CAD build for the part. Positions are in the model's coordinates, mm. A direction names the side the tool comes from. Coordinates: 2 decimals unless noted, no trailing zeros. Answer in a Markdown table with one row per item. Add a question column.
Q1. Drill centre lines: line 1 along Y through (x, z) = (-4.5, 24); line 2 along Y through (x, z) = (6, 70); line 3 along X through (y, z) = (-6, 15). Where is each one in solid material? Low to high. Write a range as from..to.
Q2. 3-axis set-ups, long thin cutter, end or side, ignore diameter. For faces 1 (the cylindrical face through (-20, -15, 40)), 2 (the cylindrical face through (0, 15, 30)), 3 (the cylindrical face through (0, -15, 30)), 4 (the cylindrical face through (-10, 0, 13)): which of +Z, -Z, +X, -X, +Y, -Y reach the whole face in a straight line?
Q3. Pin check, flat tips, straight feed: pin 1 (2 mm diameter, centred on y = 0, z = 53.5, fed in from -X); pin 2 (1 mm diameter, centred on y = 10, z = 56, fed in from -X); pin 3 (5 mm diameter, centred on y = -18.5, z = 54, fed in from -X). Stop position of each tip, or through.
```python
from build123d import *

# Parameters (mm, degrees)
F0_R         = 10
F1_DEPTH     = 25
F2_W         = 50
F2_H         = 50
F3_DEPTH     = 50
F4_T1_DEPTH  = 87.4998500005
F4_T3_DEPTH  = 0.0002
F4_T5_DEPTH  = 0.0002
F4_S9_W      = 25.5
F4_S9_H      = 25.5
F4_T10_DEPTH = 25.5
F4_S15_W     = 25.5
F4_S15_H     = 25.5
F4_T16_DEPTH = 25.5
F4_S21_W     = 25.5
F4_S21_H     = 25.5
F4_T22_DEPTH = 25.5
F4_S27_W     = 25.5
F4_S27_H     = 25.5
F4_T28_DEPTH = 25.5
F4_T34_DEPTH = 174.999500001
F4_S35_R     = 10
F4_T36_DEPTH = 91
F4_T40_DEPTH = 174.999500001
F4_S41_R     = 10
F4_T42_DEPTH = 91


# Not quite as in the source:
# - a fillet or chamfer that OpenCascade refuses, or shapes differently, is made with other operations: its cross-section is extruded or revolved along the edge and cut away or added


with BuildPart() as f1:
    # F0 (on Top) → F1 (new body)
    with BuildSketch(Plane.XY):
        Circle(F0_R)
    extrude(amount=F1_DEPTH)

    # F2 (on face) → F3 (join)
    with BuildSketch(Plane.XY.offset(25)):
        Rectangle(F2_W, F2_H)
    extrude(amount=F3_DEPTH)

    # F4: fillet of radius 25 on 10 edges, made by hand

    # F4_s2 → F4_t1 (cut)
    with BuildSketch(Plane.XY.offset(-37.4997500005)):
        with BuildLine():
            ThreePointArc((-0.0001, -25.0001), (-17.6777695297, -17.6777695297), (-25.0001, -0.0001))
            Line((-25.0001, -0.0001), (-25.5001, -0.0001))
            ThreePointArc((-25.5001, -0.0001), (-25.5, -12.50005), (-25.5, -25))
            Line((-25.5, -25), (-25, -25.5))
            ThreePointArc((-25, -25.5), (-12.50005, -25.5), (-0.0001, -25.5001))
            Line((-0.0001, -25.5001), (-0.0001, -25.0001))
        make_face()
        with BuildLine():
            ThreePointArc((25.0001, -0.0001), (17.6777695297, -17.6777695297), (0.0001, -25.0001))
            Line((0.0001, -25.0001), (0.0001, -25.5001))
            ThreePointArc((0.0001, -25.5001), (12.50005, -25.5), (25, -25.5))
            Line((25, -25.5), (25.5, -25))
            ThreePointArc((25.5, -25), (25.5, -12.50005), (25.5001, -0.0001))
            Line((25.5001, -0.0001), (25.0001, -0.0001))
        make_face()
        with BuildLine():
            ThreePointArc((25.0001, 0.0001), (17.6777695297, 17.6777695297), (0.0001, 25.0001))
            Line((0.0001, 25.0001), (0.0001, 25.5001))
            ThreePointArc((0.0001, 25.5001), (12.50005, 25.5), (25, 25.5))
            Line((25, 25.5), (25.5, 25))
            ThreePointArc((25.5, 25), (25.5, 12.50005), (25.5001, 0.0001))
            Line((25.5001, 0.0001), (25.0001, 0.0001))
        make_face()
        with BuildLine():
            ThreePointArc((-0.0001, 25.0001), (-17.6777695297, 17.6777695297), (-25.0001, 0.0001))
            Line((-25.0001, 0.0001), (-25.5001, 0.0001))
            ThreePointArc((-25.5001, 0.0001), (-25.5, 12.50005), (-25.5, 25))
            Line((-25.5, 25), (-25, 25.5))
            ThreePointArc((-25, 25.5), (-12.50005, 25.5), (-0.0001, 25.5001))
            Line((-0.0001, 25.5001), (-0.0001, 25.0001))
        make_face()
    extrude(amount=F4_T1_DEPTH, mode=Mode.SUBTRACT)

    # F4_s4 → F4_t3 (cut)
    with BuildSketch(Plane.YZ.offset(-0.0001)):
        with BuildLine():
            ThreePointArc((-25.0001, 50.0001), (-17.6777695297, 67.6777695297), (-0.0001, 75.0001))
            Line((-0.0001, 75.0001), (-0.0001, 75.5001))
            ThreePointArc((-0.0001, 75.5001), (-12.50005, 75.5), (-25, 75.5))
            Line((-25, 75.5), (-25.5, 75))
            ThreePointArc((-25.5, 75), (-25.5, 62.50005), (-25.5001, 50.0001))
            Line((-25.5001, 50.0001), (-25.0001, 50.0001))
        make_face()
        with BuildLine():
            ThreePointArc((25.0001, 50.0001), (17.6777695297, 67.6777695297), (0.0001, 75.0001))
            Line((0.0001, 75.0001), (0.0001, 75.5001))
            ThreePointArc((0.0001, 75.5001), (12.50005, 75.5), (25, 75.5))
            Line((25, 75.5), (25.5, 75))
            ThreePointArc((25.5, 75), (25.5, 62.50005), (25.5001, 50.0001))
            Line((25.5001, 50.0001), (25.0001, 50.0001))
        make_face()
    extrude(amount=F4_T3_DEPTH, mode=Mode.SUBTRACT)

    # F4_s6 → F4_t5 (cut)
    with BuildSketch(Plane.XZ.offset(-0.0001)):
        with BuildLine():
            ThreePointArc((25.0001, 50.0001), (17.6777695297, 67.6777695297), (0.0001, 75.0001))
            Line((0.0001, 75.0001), (0.0001, 75.5001))
            ThreePointArc((0.0001, 75.5001), (12.50005, 75.5), (25, 75.5))
            Line((25, 75.5), (25.5, 75))
            ThreePointArc((25.5, 75), (25.5, 62.50005), (25.5001, 50.0001))
            Line((25.5001, 50.0001), (25.0001, 50.0001))
        make_face()
        with BuildLine():
            ThreePointArc((-0.0001, 75.0001), (-17.6777695297, 67.6777695297), (-25.0001, 50.0001))
            Line((-25.0001, 50.0001), (-25.5001, 50.0001))
            ThreePointArc((-25.5001, 50.0001), (-25.5, 62.50005), (-25.5, 75))
            Line((-25.5, 75), (-25, 75.5))
            ThreePointArc((-25, 75.5), (-12.50005, 75.5), (-0.0001, 75.5001))
            Line((-0.0001, 75.5001), (-0.0001, 75.0001))
        make_face()
    extrude(amount=F4_T5_DEPTH, mode=Mode.SUBTRACT)


with BuildPart() as f4_tool8:
    # F4_s9 → F4_t10 (new body)
    with BuildSketch(Plane.XZ.offset(0.0001)):
        with Locations((-12.7501, 62.7501)):
            Rectangle(F4_S9_W, F4_S9_H)
    extrude(amount=F4_T10_DEPTH)

    # F4_s11 → F4_t12 (revolve, cut)
    with BuildSketch(Plane(origin=(-0.0001, -0.0001, 50.0001), x_dir=(0.7071067812, 0, -0.7071067812), z_dir=(-0.7071067812, 0, -0.7071067812))):
        with BuildLine():
            ThreePointArc((0, -25), (25, 0), (0, 25))
            Line((0, 25), (0, -25))
        make_face()
    revolve(axis=Axis((-0.0001, -0.0001, 50.0001), (0, -1, 0)), mode=Mode.SUBTRACT)


with BuildPart() as f1_1:
    add(f1.part)

    # F4_t7: cut F4_tool8
    add(f4_tool8.part, mode=Mode.SUBTRACT)


with BuildPart() as f4_tool14:
    # F4_s15 → F4_t16 (new body)
    with BuildSketch(Plane.YZ.offset(0.0001)):
        with Locations((-12.7501, 62.7501)):
            Rectangle(F4_S15_W, F4_S15_H)
    extrude(amount=F4_T16_DEPTH)

    # F4_s17 → F4_t18 (revolve, cut)
    with BuildSketch(Plane(origin=(0.0001, -0.0001, 50.0001), x_dir=(0, 0.7071067812, -0.7071067812), z_dir=(0, -0.7071067812, -0.7071067812))):
        with BuildLine():
            ThreePointArc((0, -25), (25, 0), (0, 25))
            Line((0, 25), (0, -25))
        make_face()
    revolve(axis=Axis((0.0001, -0.0001, 50.0001), (1, 0, 0)), mode=Mode.SUBTRACT)


with BuildPart() as f1_2:
    add(f1_1.part)

    # F4_t13: cut F4_tool14
    add(f4_tool14.part, mode=Mode.SUBTRACT)


with BuildPart() as f4_tool20:
    # F4_s21 → F4_t22 (new body)
    with BuildSketch(Plane.YZ.offset(0.0001)):
        with Locations((12.7501, 62.7501)):
            Rectangle(F4_S21_W, F4_S21_H)
    extrude(amount=F4_T22_DEPTH)

    # F4_s23 → F4_t24 (revolve, cut)
    with BuildSketch(Plane(origin=(0.0001, 0.0001, 50.0001), x_dir=(0, -0.7071067812, -0.7071067812), z_dir=(0, -0.7071067812, 0.7071067812))):
        with BuildLine():
            ThreePointArc((0, -25), (25, 0), (0, 25))
            Line((0, 25), (0, -25))
        make_face()
    revolve(axis=Axis((0.0001, 0.0001, 50.0001), (1, 0, 0)), mode=Mode.SUBTRACT)


with BuildPart() as f1_3:
    add(f1_2.part)

    # F4_t19: cut F4_tool20
    add(f4_tool20.part, mode=Mode.SUBTRACT)


with BuildPart() as f4_tool26:
    # F4_s27 → F4_t28 (new body)
    with BuildSketch(Plane.XZ.offset(-0.0001)):
        with Locations((-12.7501, 62.7501)):
            Rectangle(F4_S27_W, F4_S27_H)
    extrude(amount=-F4_T28_DEPTH)

    # F4_s29 → F4_t30 (revolve, cut)
    with BuildSketch(Plane(origin=(-0.0001, 0.0001, 50.0001), x_dir=(0.7071067812, 0, -0.7071067812), z_dir=(0.7071067812, 0, 0.7071067812))):
        with BuildLine():
            ThreePointArc((0, -25), (25, 0), (0, 25))
            Line((0, 25), (0, -25))
        make_face()
    revolve(axis=Axis((-0.0001, 0.0001, 50.0001), (0, 1, 0)), mode=Mode.SUBTRACT)


with BuildPart() as f1_4:
    add(f1_3.part)

    # F4_t25: cut F4_tool26
    add(f4_tool26.part, mode=Mode.SUBTRACT)


with BuildPart() as f4_tool32:
    # F4_s33 → F4_t34 (new body)
    with BuildSketch(Plane.YZ.offset(-87.4997500005)):
        with BuildLine():
            ThreePointArc((-25.0001, 49.9999), (-17.6777695297, 32.3222304703), (-0.0001, 24.9999))
            Line((-0.0001, 24.9999), (-0.0001, 24.4999))
            ThreePointArc((-0.0001, 24.4999), (-12.50005, 24.5), (-25, 24.5))
            Line((-25, 24.5), (-25.5, 25))
            ThreePointArc((-25.5, 25), (-25.5, 37.49995), (-25.5001, 49.9999))
            Line((-25.5001, 49.9999), (-25.0001, 49.9999))
        make_face()
    extrude(amount=F4_T34_DEPTH)

    # F4_s35 → F4_t36 (cut, symmetric)
    with BuildSketch(Plane.XY.offset(37.2)):
        Circle(F4_S35_R)
    extrude(amount=F4_T36_DEPTH, both=True, mode=Mode.SUBTRACT)


with BuildPart() as f1_5:
    add(f1_4.part)

    # F4_t31: cut F4_tool32
    add(f4_tool32.part, mode=Mode.SUBTRACT)


with BuildPart() as f4_tool38:
    # F4_s39 → F4_t40 (new body)
    with BuildSketch(Plane.YZ.offset(87.4997500005)):
        with BuildLine():
            ThreePointArc((25.0001, 49.9999), (17.6777695297, 32.3222304703), (0.0001, 24.9999))
            Line((0.0001, 24.9999), (0.0001, 24.4999))
            ThreePointArc((0.0001, 24.4999), (12.50005, 24.5), (25, 24.5))
            Line((25, 24.5), (25.5, 25))
            ThreePointArc((25.5, 25), (25.5, 37.49995), (25.5001, 49.9999))
            Line((25.5001, 49.9999), (25.0001, 49.9999))
        make_face()
    extrude(amount=-F4_T40_DEPTH)

    # F4_s41 → F4_t42 (cut, symmetric)
    with BuildSketch(Plane.XY.offset(37.2)):
        Circle(F4_S41_R)
    extrude(amount=F4_T42_DEPTH, both=True, mode=Mode.SUBTRACT)


with BuildPart() as f1_6:
    add(f1_5.part)

    # F4_t37: cut F4_tool38
    add(f4_tool38.part, mode=Mode.SUBTRACT)


solid = f1_6.part
```
Checked values:
| question | item | result |
|---|---|---|
| 1 | line 1 | y = -8.93..8.93 |
| 1 | line 2 | y = -13.75..13.75 |
| 1 | line 3 | x = -8..8 |
| 2 | face 1 | +Z, -Z, -X, -Y |
| 2 | face 2 | -Z, +Y |
| 2 | face 3 | -Z, -Y |
| 2 | face 4 | -Z |
| 3 | pin 1 | stops at x = -24.87 |
| 3 | pin 2 | stops at x = -22.37 |
| 3 | pin 3 | stops at x = -18.85 |
